```python
from build123d import *

# Parameters (mm, degrees)
SKETCH_2_W           = 8.167130209
SKETCH_2_H           = 10
SKETCH_2_R           = 1.75
EXTRUDE_1_DEPTH      = 1.5
EXTRUDE_1_DEPTH_BACK = 1.5


with BuildPart() as part:
    # Sketch 1 → Revolve 1 (revolve)
    with BuildSketch(Plane(origin=(0, 0, 0), x_dir=(1, 0, 0), z_dir=(0, 1, 0))):
        Polygon((25.35, 72.313545186), (31.5, 72.313545186), (27.7, 64.313545186), (27.7, 38.313545186), (15.641285641, 29.17200386), (15.641285641, -1.349457697), (13.76021029, -3.686454814), (0, -3.686454814), (0, 28.127467739), (13, 28.127467739), (25.35, 38.313545186), align=None)
    revolve(axis=Axis((0, 0, 0), (0, 0, -1)))

    # Sketch 2 → Extrude 1 (add, two sides)
    with BuildSketch(Plane(origin=(0, 0, 0), x_dir=(1, 0, 0), z_dir=(0, 1, 0))) as extrude_1_sk:
        with Locations((29.266434896, 54.282588322)):
            Rectangle(SKETCH_2_W, SKETCH_2_H)
        with Locations((29.266434895, 54.282588322)):
            Circle(SKETCH_2_R, mode=Mode.SUBTRACT)
        with Locations((-29.266434896, 54.282588322)):
            Rectangle(SKETCH_2_W, SKETCH_2_H)
        with Locations((-29.266434895, 54.282588322)):
            Circle(SKETCH_2_R, mode=Mode.SUBTRACT)
    extrude(amount=EXTRUDE_1_DEPTH)
    extrude(extrude_1_sk.sketch, amount=-EXTRUDE_1_DEPTH_BACK)


solid = part.part
```
The listing builds one solid part. Answer for the finished solid, in the listing's coordinates (mm). A direction names the side the tool comes from. Round coordinates to 2 decimals unless told otherwise and drop trailing zeros. Loops run counter-clockwise (first coordinate to the right, second up) from the corner with the lowest first, then second, coordinate; pieces in that order, holes last.
Q1. Section B-B, the plane x = 0 is taken. Determine the outline of the cut face in (y, z).
Q2. Section D-D, the plane z = -16.5 is taken. Determine the outline of the cut face in (x, y).
Q3. Find the intervals of material crossed by line 1 (X direction, y = 0, z = -55); line 2 (Y direction, x = 0, z = -64), in increasing order.
Q4. For a pull along Z with two mould halves and no side action, classify faces 4 (the face through (32, -1.5, -54)), 5 (the face through (-31.015, -0.021, -54.35)), 6 (the face through (15.477, -4.874, -29.616)) as released by +Z, released by -Z, zero draft, split by the parting line, or undercut.
Q5. Which of the six approach directions +Z, -Z, +X, -X, +Y, -Y give full straight-line access (tool end or side, diameter ignored) to faces 1 (the face through (0, 0, -28.127)), 2 (the face through (-12.41, 9.52, -13.7)), 3 (the face through (-31, 0, -49.283))?
Q6. Given pin 1 Ø1 at (x, y) = (-1.5, 13.5) entering from -Z; pin 2 Ø1.5 at (y, z) = (22, -59.5) entering from -X; pin 3 Ø3 at (x, z) = (29.27, -54.28) entering from +Y; pin 4 Ø1 at (x, z) = (-12.5, -14) entering from -Y, each flat-ended and moving along its own axis, determine where each tip first touches the part or whether it passes through.
Q7. Section C-C, the plane y = 0 is taken. Count the separate pieces of the cut face and the enclosed holes in it, then the cut area to 3 significant figures.
Completed:
1. outline: (-31.5, -72.31) - (-25.35, -72.31) - (-25.35, -38.31) - (-13, -28.13) - (13, -28.13) - (25.35, -38.31) - (25.35, -72.31) - (31.5, -72.31) - (27.7, -64.31) - (27.7, -38.31) - (15.64, -29.17) - (15.64, 1.35) - (13.76, 3.69) - (-13.76, 3.69) - (-15.64, 1.35) - (-15.64, -29.17) - (-27.7, -38.31) - (-27.7, -64.31) - close
2. outline: circle Ø31.28 at (0, 0)
3. line 1: x = -33.35 to -30.86, -27.7 to -25.18, 25.18 to 27.7, 30.86 to 33.35
3. line 2: y = -27.7 to -25.35, 25.35 to 27.7
4. face 4: zero draft
4. face 5: undercut
4. face 6: released by +Z
5. face 1: -Z
5. face 2: +Z
5. face 3: +Z, -X, +Y, -Y
6. pin 1: stops at z = -29.02
6. pin 2: stops at x = -17.77
6. pin 3: passes through
6. pin 4: stops at y = -10.03
7. separate pieces: 1
7. enclosed holes: 2
7. area: 1,320 mm2
